Here's how the part is built. I have some questions about the finished solid (model axes, mm). A direction names the side the tool comes from. Round coordinates to 2 decimals unless told otherwise and drop trailing zeros. Write each loop counter-clockwise with the first axis right and the second up, starting at its lowest first coordinate (ties: lowest second). Pieces come first, ordered by that corner, then holes. Notation, with made-up numbers: (31.5, -0.5) -> (63.5, -0.5) arc R8 ccw to (63.5, 10.5) -> close; hole circle Ø4 at (85.5, -4.75). An arc over 180 degrees is marked (long way). Answer as CSV lines item,"result".
```python
from build123d import *

# Parameters (mm, degrees)
BOSS_EXTRUDE1_DEPTH = 5
SKETCH2_R           = 2.35
CUT_EXTRUDE1_DEPTH  = 3
SKETCH3_W           = 32
SKETCH3_H           = 15.5
SKETCH3_W_2         = 5
SKETCH3_H_2         = 10
BOSS_EXTRUDE2_DEPTH = 2.4
SKETCH4_W           = 32
SKETCH4_H           = 15.5
SKETCH4_W_2         = 24
SKETCH4_H_2         = 11.7
BOSS_EXTRUDE3_DEPTH = 15.1
SKETCH6_R           = 1.125
CUT_EXTRUDE2_DEPTH  = 8


with BuildPart() as part:
    # Sketch1 → Boss-Extrude1 (new body)
    with BuildSketch(Plane.XY):
        with BuildLine():
            Line((0, 5), (20.9, 5))
            Line((20.9, 5), (20.9, -5))
            Line((20.9, -5), (0, -5))
            ThreePointArc((0, -5), (-5, 0), (0, 5))
        make_face()
    extrude(amount=BOSS_EXTRUDE1_DEPTH)

    # Sketch2 → Cut-Extrude1 (cut)
    with BuildSketch(Plane(origin=(0, 0, 0), x_dir=(-1, 0, 0), z_dir=(0, 0, -1))):
        Circle(SKETCH2_R)
    extrude(amount=-CUT_EXTRUDE1_DEPTH, mode=Mode.SUBTRACT)

    # Sketch3 → Boss-Extrude2 (add)
    with BuildSketch(Plane(origin=(20.9, 0, 0), x_dir=(0, 0, -1), z_dir=(1, 0, 0))):
        with Locations((8.15, 0)):
            Rectangle(SKETCH3_W, SKETCH3_H)
        with Locations((-2.5, 0)):
            Rectangle(SKETCH3_W_2, SKETCH3_H_2, mode=Mode.SUBTRACT)
    extrude(amount=-BOSS_EXTRUDE2_DEPTH)

    # Sketch4 → Boss-Extrude3 (add)
    with BuildSketch(Plane(origin=(20.9, 0, 0), x_dir=(0, 0, -1), z_dir=(1, 0, 0))):
        with Locations((8.15, 0)):
            Rectangle(SKETCH4_W, SKETCH4_H)
        with Locations((8.15, 0)):
            Rectangle(SKETCH4_W_2, SKETCH4_H_2, mode=Mode.SUBTRACT)
    extrude(amount=BOSS_EXTRUDE3_DEPTH)

    # Sketch6 → Cut-Extrude2 (cut)
    with BuildSketch(Plane(origin=(36, 0, 0), x_dir=(0, 0, -1), z_dir=(1, 0, 0))):
        with Locations((-5.8, 0)):
            Circle(SKETCH6_R)
        with Locations((22.1, 0)):
            Circle(SKETCH6_R)
    extrude(amount=-CUT_EXTRUDE2_DEPTH, mode=Mode.SUBTRACT)


solid = part.part
```
1. Suppose I cut it at D-D on z = -19. Please give me the cut outline in (x, y).
Numbers:
outline,"(18.5, -7.75) -> (36, -7.75) -> (36, -5.85) -> (20.9, -5.85) -> (20.9, 5.85) -> (36, 5.85) -> (36, 7.75) -> (18.5, 7.75) -> close"
2. Suppose I cut it at C-C on y = -4. Please give me the cut outline in (x, z), and give its area (3 significant figures).
Numbers:
outline,"(-3, 0) -> (18.5, 0) -> (18.5, -24.15) -> (36, -24.15) -> (36, -20.15) -> (20.9, -20.15) -> (20.9, 3.85) -> (36, 3.85) -> (36, 7.85) -> (18.5, 7.85) -> (18.5, 5) -> (-3, 5) -> close"
area,"305 mm^2"
3. On a 3-axis mill with a long thin cutter (end or side, diameter ignored), from which of +Z, -Z, +X, -X, +Y, -Y can I reach the whole of each face in a straight line? I mean faces 5 (the face through (0.509, -2.294, 1.479)), 6 (the face through (7, 0, 0)), 7 (the face through (9, -5, 2)), 8 (the face through (7, 0, 5)), 9 (the face through (28, -5.85, -8)). Say none if no direction works.
Numbers:
face 5,"-Z"
face 6,"-Z, -X, +Y, -Y"
face 7,"+Z, -Z, -X, -Y"
face 8,"+Z, -X, +Y, -Y"
face 9,"+X"
4. Suppose I cut it at A-A on z = 1. Please give me the cut outline in (x, y), and give its area (4 significant figures).
Numbers:
outline,"(0, -5) -> (18.5, -5) -> (18.5, -7.75) -> (36, -7.75) -> (36, -5.85) -> (20.9, -5.85) -> (20.9, 5.85) -> (36, 5.85) -> (36, 7.75) -> (18.5, 7.75) -> (18.5, 5) -> (0, 5) arc R5 ccw to start; hole circle Ø4.7 at (0, 0)"
area,"301.5 mm^2"
5. If we mould it in two halves opening along Z, with no side actions, what happens to faces 1 (the face through (28, 0, -22)), 2 (the face through (9, 5, 2)), 3 (the face through (27, 0, -24.15)), 4 (the face through (28, 0, -20.15))? For each: released by +Z, released by -Z, zero draft, split by the parting line, or undercut.
Numbers:
face 1,"undercut"
face 2,"zero draft"
face 3,"released by -Z"
face 4,"undercut"
6. If I drill on line 1 (Y direction, x = 25.5, z = -2); line 2 (Y direction, x = 30.25, z = -22.1) (3 decimals); line 3 (Z direction, x = 26.5, y = -1.75), over which ranges is the centre line in solid material (lowest first)?
Numbers:
line 1,"y = -7.75 to -5.85, 5.85 to 7.75"
line 2,"y = -7.75 to -1.125, 1.125 to 7.75"
line 3,"z = -24.15 to -20.15, 3.85 to 7.85"
7. Suppose I cut it at B-B on x = 33.5. Please give me the cut outline in (y, z) (3 decimals).
Numbers:
outline,"(-7.75, -24.15) -> (7.75, -24.15) -> (7.75, 7.85) -> (-7.75, 7.85) -> close; hole (-5.85, -20.15) -> (5.85, -20.15) -> (5.85, 3.85) -> (-5.85, 3.85) -> close; hole circle Ø2.25 at (0, -22.1); hole circle Ø2.25 at (0, 5.8)"
8. For pin 1 Ø5 at (x, y) = (15, 3) entering from -Z; pin 2 Ø1.5 at (x, z) = (3, 1.5) entering from +Y; pin 3 Ø5 at (y, z) = (-0.5, -4) entering from +X; pin 4 Ø3.5 at (y, z) = (0, 5.8) entering from +X, each with a flat end and sliding along its axis, tell me the tip position at first contact or that it passes through.
Numbers:
pin 1,"stops at z = 0"
pin 2,"stops at y = 5"
pin 3,"stops at x = 20.9"
pin 4,"stops at x = 36"
